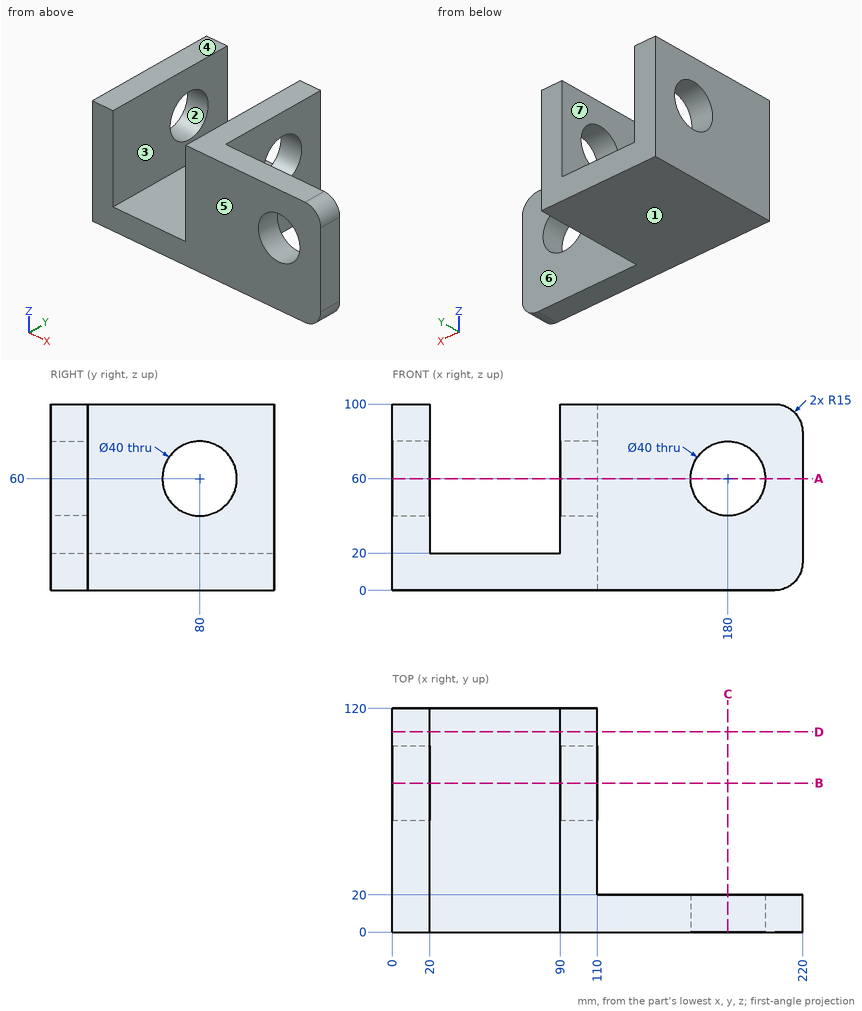
Here's the drawing with two shaded views (mm, measured from the low corner). I have some questions. A direction names the side the tool comes from. Coordinates: 2 decimals unless noted, no trailing zeros. Loops run counter-clockwise (first coordinate to the right, second up) from the corner with the lowest first, then second, coordinate; pieces in that order, holes last. Notation, with made-up numbers: (69.5, 43.5) -> (80.5, 43.5) arc R26 ccw to (80.5, 59.5) -> close; hole circle Ø10 at (-3, -11.5). An arc over 180 degrees is marked (long way). Put each result on its own line as item: value. Start each with the question number.
Q1. I want a section at C-C (x = 180). Write out the boundary of the cut face in (y, z).
Q2. If I drill on line 1 (X direction, y = 28, z = 63.5); line 2 (Y direction, x = 7, z = 60); line 3 (Z direction, x = 103.5, y = 80), over which ranges is the centre line in solid material (lowest first)? Write a range as [from, to].
Q3. I want a section at B-B (y = 80). Write out the boundary of the cut face in (x, z).
Q4. I want a section at D-D (y = 107.5). Write out the boundary of the cut face in (x, z), plus the area to 3 significant figures.
Q5. For the marked faces 5, 6 and 7, which set-ups out of +Z, -Z, +X, -X, +Y, -Y let a thin tool reach every point of the face, with its end or its side?
Q6. Thinking about a two-plate mould opening in Z: for the marked faces 1, 2, 3 and 4, which applies, pulls with the +Z half, pulls with the -Z half, needs draft (parallel to the pull), parting line crosses it, or undercut?
Q7. I'm going to push flat-ended pins straight in: P1, Ø1, axis at x = 56, y = 16, coming from the +Z side; P2, Ø1, axis at y = 63.5, z = 11.5, coming from the +X side; P3, Ø10, axis at x = 134, z = 73, coming from the -Y side. Where does each tip first touch, or does it pass through?
Q8. I want a section at A-A (z = 60). Write out the boundary of the cut face in (x, y).
Taken from the geometry:
1. outline: (0, 0) -> (20, 0) -> (20, 40) -> (0, 40) -> close; (0, 80) -> (20, 80) -> (20, 100) -> (0, 100) -> close
2. line 1: x = [0, 20], [90, 110]
2. line 2: y = [0, 60], [100, 120]
2. line 3: z = [0, 40], [80, 100]
3. outline: (0, 0) -> (110, 0) -> (110, 40) -> (90, 40) -> (90, 20) -> (20, 20) -> (20, 40) -> (0, 40) -> close; (0, 80) -> (20, 80) -> (20, 100) -> (0, 100) -> close; (90, 80) -> (110, 80) -> (110, 100) -> (90, 100) -> close
4. outline: (0, 0) -> (110, 0) -> (110, 100) -> (90, 100) -> (90, 20) -> (20, 20) -> (20, 100) -> (0, 100) -> close
4. area: 5,400 mm2
5. face 5: +Z, -Z, +X, -X, -Y
5. face 6: +Z, -Z, +X, +Y
5. face 7: +Z, +Y, -Y
6. face 1: pulls with the -Z half
6. face 2: undercut
6. face 3: needs draft
6. face 4: pulls with the +Z half
7. P1: stops at z = 20
7. P2: stops at x = 110
7. P3: stops at y = 0
8. outline: (0, 0) -> (20, 0) -> (20, 60) -> (0, 60) -> close; (0, 100) -> (20, 100) -> (20, 120) -> (0, 120) -> close; (90, 0) -> (160, 0) -> (160, 20) -> (110, 20) -> (110, 60) -> (90, 60) -> close; (90, 100) -> (110, 100) -> (110, 120) -> (90, 120) -> close; (200, 0) -> (220, 0) -> (220, 20) -> (200, 20) -> close
